Study the drawing (mm; zero at the part's minimum x, y, z) and answer. Give positions to 0.01 mm unless a question says otherwise; leave off trailing zeros. Put each result on its own line as item: value. Start each with the question number.
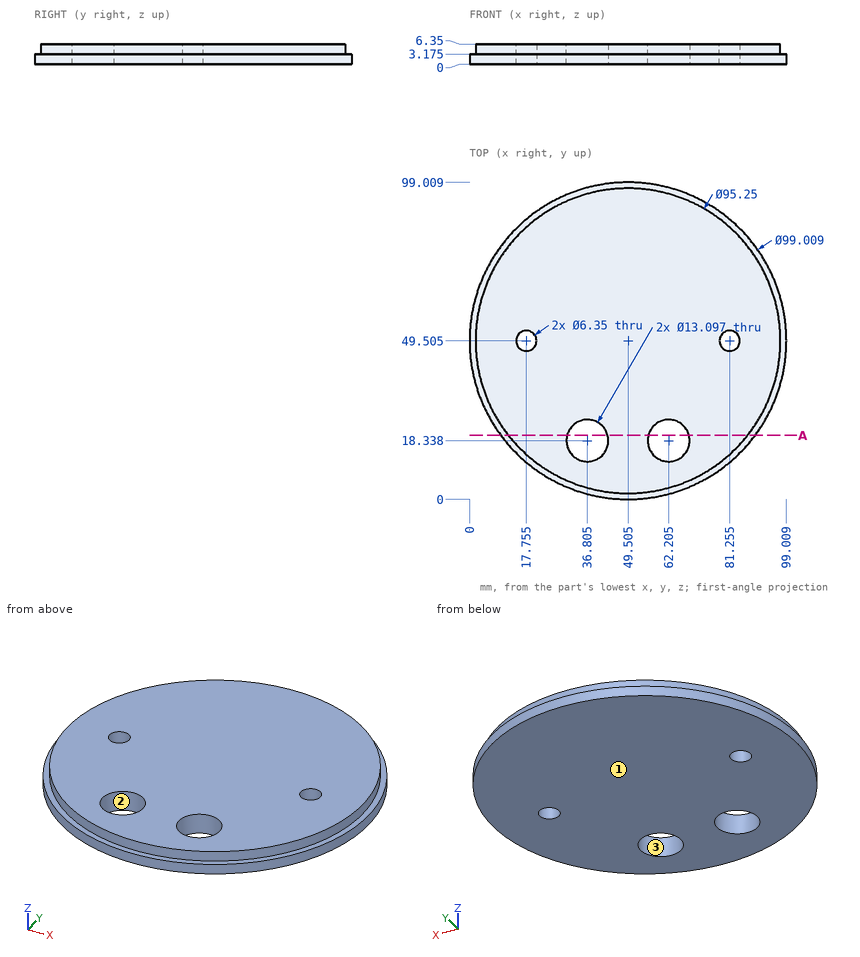
1) A cutting plane is placed at A-A on y = 20. State how many separate pieces and enclosed holes the cut face has, and give its area (3 significant figures).
2) Straight lines are drawn through the part: line 1 (X direction, y = 47, z = 2.5) (1 decimal); line 2 (X direction, y = 21.5, z = 2.5) (1 decimal); line 3 (Y direction, x = 19, z = 2) (1 decimal). For each, find the intervals that lie inside material, in ascending order. Write a range as [from, to].
3) Each of these flat-tipped pins is pushed along its axis until it touches: pin 1 Ø1 at (x, z) = (25, 4.5) entering from +Y; pin 2 Ø1 at (x, z) = (34.5, 4) entering from +Y; pin 3 Ø3 at (y, z) = (69.5, 2) entering from +X (1 decimal). Where does it stop, or does it pass through?
4) For a pull along Y with two mould halves and no side action, classify the marked faces 1, 2 and 3 as pulls with the +Y half, pulls with the -Y half, needs draft (parallel to the pull), parting line crosses it, or undercut.
Results found:
1. separate pieces: 3
1. enclosed holes: 0
1. area: 329 mm²
2. line 1: x = [0.1, 15.8], [19.7, 79.3], [83.2, 98.9]
2. line 2: x = [8.7, 31.1], [42.5, 56.5], [67.9, 90.3]
2. line 3: y = [10.5, 46.6], [52.4, 88.5]
3. pin 1: stops at y = 90.64
3. pin 2: stops at y = 94.87
3. pin 3: stops at x = 95.4
4. face 1: needs draft
4. face 2: undercut
4. face 3: undercut
